from build123d import *

# Parameters (mm, degrees)
F0_W     = 50
F0_H     = 50
F1_DEPTH = 10
F3_DEPTH = 10
F5_DEPTH = 10
F7_D     = 5.5
F8_D     = 3


with BuildPart() as f1:
    # F0 (on Top) → F1 (new body)
    with BuildSketch(Plane.XY):
        Rectangle(F0_W, F0_H)
    extrude(amount=F1_DEPTH)

    # F2 (on Top) → F3 (cut, through all)
    with BuildSketch(Plane.XY):
        with BuildLine():
            Line((-4.8989794856, -1), (-9.9498743711, -1))
            ThreePointArc((-9.9498743711, -1), (0, -10), (9.9498743711, -1))
            Line((9.9498743711, -1), (4.8989794856, -1))
            ThreePointArc((4.8989794856, -1), (0, -5), (-4.8989794856, -1))
        make_face()
        with BuildLine():
            ThreePointArc((9.9498743711, 1), (0, 10), (-9.9498743711, 1))
            Line((-9.9498743711, 1), (-4.8989794856, 1))
            ThreePointArc((-4.8989794856, 1), (0, 5), (4.8989794856, 1))
            Line((4.8989794856, 1), (9.9498743711, 1))
        make_face()
    extrude(amount=F3_DEPTH, mode=Mode.SUBTRACT)

    # F4 (on Top) → F5 (join)
    with BuildSketch(Plane.XY):
        Polygon((2, 9), (-2, 9), (-2, 4.8284271247), (2, 0.8284271247), align=None)
        Polygon((2, 0.8284271247), (-2, 4.8284271247), (-2, -0.8284271247), (2, -4.8284271247), align=None)
        Polygon((-2, -0.8284271247), (-2, 4.8284271247), (-4.9497474683, 7.7781745931), (-7.7781745931, 4.9497474683), align=None)
        Polygon((7.7781745931, -4.9497474683), (2, 0.8284271247), (2, -4.8284271247), (4.9497474683, -7.7781745931), align=None)
        Polygon((2, -4.8284271247), (-2, -0.8284271247), (-2, -9), (2, -9), align=None)
    extrude(amount=F5_DEPTH)

    # F7 (through all)
    with Locations(Plane(origin=(0, 0, 0), x_dir=(1, 0, 0), z_dir=(0, 0, -1))):
        with Locations((0, 0)):
            Hole(F7_D / 2)

    # F8 (through all)
    with Locations(Plane(origin=(0, 0, 0), x_dir=(1, 0, 0), z_dir=(0, 0, -1))):
        with Locations((-6.7175144213, -6.7175144213), (0, -10), (0, 9.5), (6.7175144213, 6.7175144213)):
            Hole(F8_D / 2)


solid = f1.part
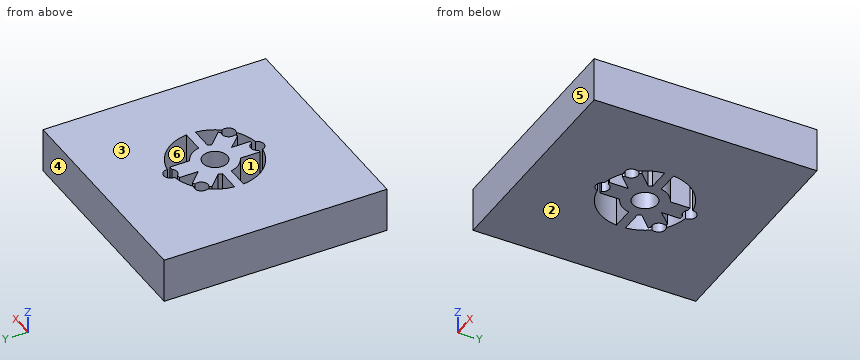
Could you check a few things on this model? Use its own coordinates, in mm. Face numbers are marked on the shaded views. A direction names the side the tool comes from. Round coordinates to 2 decimals unless told otherwise and drop trailing zeros. Write each loop counter-clockwise with the first axis right and the second up, starting at its lowest first coordinate (ties: lowest second). Pieces come first, ordered by that corner, then holes. Notation, with made-up numbers: (-8, 55) -> (34, 55) arc R14 ccw to (34, 63) -> close; hole circle Ø8 at (-18, -32.75). An arc over 180 degrees is marked (long way). Use a Markdown table: item, result.
1. We'd pull the mould along Y, two halves only. Please class the marked faces 3, 4, 5 and 6: +Y half, -Y half, draft (parallel to the pull), parting line (faces both ways), or undercut.
Answer key:
| item | result |
|---|---|
| face 3 | draft |
| face 4 | +Y half |
| face 5 | -Y half |
| face 6 | undercut |
2. If we section it at C-C (z = 4.25): State how many separate pieces and enclosed holes the cut face has, then the cut area to 3 significant figures.
Answer key:
| item | result |
|---|---|
| separate pieces | 1 |
| enclosed holes | 3 |
| area | 2,310 mm^2 |
3. If we section it at A-A (y = 0): List the corners of the cut face in (x, z) for me, then the cut area to 3 significant figures.
Answer key:
| item | result |
|---|---|
| outline | (-25, 0) -> (-2.75, 0) -> (-2.75, 10) -> (-25, 10) -> close; (2.75, 0) -> (25, 0) -> (25, 10) -> (2.75, 10) -> close |
| area | 445 mm^2 |
4. Please list where these lines run through material, in increasing order: probe 1 along Y at (x, z) = (0, 4); probe 2 along X at (y, z) = (-7.5, 5.75); probe 3 along X at (y, z) = (-4, 9.5).
Answer key:
| item | result |
|---|---|
| probe 1 | y = -25 to -11, -8 to -2.75, 2.75 to 8.5, 11.5 to 25 |
| probe 2 | x = -25 to -6.61, -2 to 2, 4.67 to 5.23, 8 to 25 |
| probe 3 | x = -25 to -9.17, -3 to 6.83, 9.17 to 25 |
5. If we section it at B-B (x = 0): List the corners of the cut face in (y, z) for me.
Answer key:
| item | result |
|---|---|
| outline | (-25, 0) -> (-11, 0) -> (-11, 10) -> (-25, 10) -> close; (-8, 0) -> (-2.75, 0) -> (-2.75, 10) -> (-8, 10) -> close; (2.75, 0) -> (8.5, 0) -> (8.5, 10) -> (2.75, 10) -> close; (11.5, 0) -> (25, 0) -> (25, 10) -> (11.5, 10) -> close |
6. Which directions (+Z, -Z, +X, -X, +Y, -Y) give clear straight access to the entire face, cutting with the end or side of a thin tool? Please do the marked faces 1 and 2.
Answer key:
| item | result |
|---|---|
| face 1 | +Z, -Z |
| face 2 | -Z, +X, -X, +Y, -Y |
